Here's how the part is built. I have some questions about the finished solid (model axes, mm). A direction names the side the tool comes from. Give positions to 0.01 mm unless a question says otherwise; leave off trailing zeros. Loops run counter-clockwise (first coordinate to the right, second up) from the corner with the lowest first, then second, coordinate; pieces in that order, holes last. Notation, with made-up numbers: M 72,-6 L 115,-6 A23 ccw 115,33 Z; hole C -38.75,-20 d4. An arc over 180 degrees is marked long. Write item = value, one per line. Start each with the question number.
```python
from build123d import *

# Parameters (mm, degrees)
BOSS_EXTRUDE2_DEPTH = 3.175


with BuildPart() as part:
    # Sketch1 → Boss-Extrude2 (new body, symmetric)
    with BuildSketch(Plane.XY):
        with BuildLine():
            ThreePointArc((-21.30491262, -43.851351885), (32.502343983, -30.45576299), (9.776598146, 20.122919685))
            ThreePointArc((9.776598146, 20.122919685), (1.347485848, 38.882849469), (21.30491262, 43.851351885))
            ThreePointArc((21.30491262, 43.851351885), (-32.502343983, 30.45576299), (-9.776598146, -20.122919685))
            ThreePointArc((-9.776598146, -20.122919685), (-1.347485848, -38.882849469), (-21.30491262, -43.851351885))
        make_face()
        Polygon((0, 14.664696837), (-12.7, 7.332348419), (-12.7, -7.332348419), (0, -14.664696837), (12.7, -7.332348419), (12.7, 7.332348419), align=None, mode=Mode.SUBTRACT)
    extrude(amount=BOSS_EXTRUDE2_DEPTH, both=True)


solid = part.part
```
Q1. If we section it at C-C, the plane z = 0: List the corners of the cut face in (x, y) for me.
Q2. If I drill on line 1 along Y through (x, z) = (2, 0.75); line 2 along Y through (x, z) = (-1, 1); line 3 along X through (y, z) = (9, -1.25), over which ranges is the centre line in solid material (lowest first)?
Q3. If we section it at B-B, the plane y = 12: List the corners of the cut face in (x, z) for me (3 decimals), then the cut area to 3 significant figures.
Q4. If we section it at D-D, the plane x = 18.5: List the corners of the cut face in (y, z) for me (3 decimals), then the cut area to 3 significant figures.
Q5. If we section it at A-A, the plane x = 11: List the corners of the cut face in (y, z) for me (1 decimal), then the cut area to 3 significant figures.
Q6. Will these pins go through, and if not, where does the flat tip stop? pin 1 (16 mm diameter, centred on x = -13.4, y = -33.03, fed in from +Z); pin 2 (1 mm diameter, centred on x = 7.5, z = 0.5, fed in from -Y); pin 3 (3 mm diameter, centred on y = 9.5, z = 2, fed in from -X).
Q7. On a 3-axis mill with a long thin cutter (end or side, diameter ignored), from which of +Z, -Z, +X, -X, +Y, -Y can I reach the whole of each face in a straight line? I mean faces 3 (the flat face through (6.439, 10.947, 0.044)), 4 (the flat face through (8, 12, -3.175)). Say none if no direction works.
Q8. We'd pull the mould along Y, two halves only. Please class faces 1 (the cylindrical face through (-1.21, -38.59, 0.04)), 2 (the flat face through (8, 12, 3.175)): pulls with the +Y half, pulls with the -Y half, needs draft (parallel to the pull), parting line crosses it, or undercut.
Resolved:
q1.outline = M -21.3,-43.85 A36.14 ccw long 9.78,20.12 A13.4 cw long 21.3,43.85 A36.14 ccw long -9.78,-20.12 A13.4 cw long Z; hole M -12.7,-7.33 L 0,-14.66 L 12.7,-7.33 L 12.7,7.33 L 0,14.66 L -12.7,7.33 Z
q2.line_1 = -50.74 to -13.51, 13.51 to 25.98, 40.07 to 50.74
q2.line_2 = -50.79 to -38.11, -27.95 to -14.09, 14.09 to 50.79
q2.line_3 = -35.69 to -9.81, 9.81 to 27.31
q3.outline = M -36.037,-3.175 L -4.615,-3.175 L -4.615,3.175 L -36.037,3.175 Z; M 4.615,-3.175 L 24.388,-3.175 L 24.388,3.175 L 4.615,3.175 Z
q3.area = 325 mm²
q4.outline = M -45.705,-3.175 L 16.376,-3.175 L 16.376,3.175 L -45.705,3.175 Z; M 45.422,-3.175 L 45.705,-3.175 L 45.705,3.175 L 45.422,3.175 Z
q4.area = 396 mm²
q5.outline = M -49.1,-3.2 L -8.3,-3.2 L -8.3,3.2 L -49.1,3.2 Z; M 8.3,-3.2 L 19.8,-3.2 L 19.8,3.2 L 8.3,3.2 Z; M 46.2,-3.2 L 49.1,-3.2 L 49.1,3.2 L 46.2,3.2 Z
q5.area = 350 mm²
q6.pin_1 = through
q6.pin_2 = -50.12
q6.pin_3 = -35.95
q7.face_3 = +Z, -Z
q7.face_4 = -Z, +X, -X, +Y, -Y
q8.face_1 = undercut
q8.face_2 = needs draft
